Model file for the job. Use its own axes, mm. A direction names the side the tool comes from. Give positions to 0.01 mm unless a question says otherwise; leave off trailing zeros. Order: outer loops, then holes, each group sorted by start corner. A loop starts at its lowest first (then second) coordinate and runs counter-clockwise, first axis right, second up. Notation, with made-up numbers: M 82.5,-6.5 L 110.5,-6.5 A17 ccw 110.5,20.5 Z; hole C 72.5,85 d2. An arc over 180 degrees is marked long. Return JSON: item names as keys, results as strings. Group by question number.
1. Two-plate mould, pull along X, no slides. Class faces 4 (the face through (42.9, 3.4, 23.6)), 5 (the face through (1, 5, 0)), 6 (the face through (-44.45, 4.51, 22.3)): released by +X, released by -X, zero draft, split by the parting line, or undercut.
2. Slice it at C-C on z = 0. List the corners of the cut face in (x, y).
3. Wall check: probe 1 along X at (y, z) = (2.6, 25); probe 2 along Z at (x, y) = (-41.5, 3.65); probe 3 along X at (y, z) = (4.35, 25). Give the ranges that are in metal, low to high. Write a range as [from, to].
4. 3-axis set-ups, long thin cutter, end or side, ignore diameter. For faces 1 (the face through (40.979, 4.507, -28.966)), 2 (the face through (-38.327, 1.724, 25.705)), 3 (the face through (-29.084, 2.465, -2.703)): which of +Z, -Z, +X, -X, +Y, -Y reach the whole face in a straight line?
5. Slice it at A-A on z = 25. List the corners of the cut face in (x, y).
6. Slice it at D-D on y = 2.1. Give the number of separate pieces and of enclosed holes in the cut face, then the cut area to 3 significant figures.
7. Slice it at B-B on x = -20.5. List the corners of the cut face in (y, z).
8. Pin check, flat tips, straight feed: pin 1 (2 mm diameter, centred on x = -40.5, z = -24.5, fed in from -Y); pin 2 (7.5 mm diameter, centred on x = -41.5, z = 25, fed in from +Y). Stop position of each tip, or through.
Autodesk Inventor part; units mm, degrees
ref_plane "YZ Plane" through (0, 0, 0) normal (1, 0, 0) x (0, 1, 0)
ref_plane "XZ Plane" through (0, 0, 0) normal (0, 1, 0) x (-1, 0, 0)
ref_plane "XY Plane" through (0, 0, 0) normal (0, 0, 1) x (1, 0, 0)
sketch "Sketch1" plane through (0, 0, 0) normal (0, 1, 0) x (-1, 0, 0)
  line L0 (46.5, 30) -> (-46.5, 30)
  line L1 (-46.5, 30) -> (-46.5, -30)
  line L2 (-46.5, -30) -> (46.5, -30)
  line L3 (46.5, -30) -> (46.5, 30)
  line L4 (46.5, 30) -> (-46.5, -30) construction
  line L5 (-46.5, 30) -> (46.5, -30) construction
  circle A0 centre (20.5, 0) radius 9
  circle A1 centre (-19.5, 0) radius 12.5
  line L6 (152.1746, 0) -> (-152.1746, 0) construction
  line L7 (0, 58.0523) -> (0, -58.0523) construction
  point P0 (0, 0)
  dimension "d0" = 93
  dimension "d1" = 18
  dimension "d2" = 25
  dimension "d3" = 26
  dimension "d4" = 60
  dimension "d5" = 27
extrude "Extrusion1" add sketch "Sketch1" along normal blind 5
sketch "Sketch2" plane through (0, 0, 0) normal (0, -1, 0) x (1, 0, 0)
  line L0 (41.5, 25) -> (-41.5, 25) construction
  line L1 (-41.5, 25) -> (-41.5, -25) construction
  line L2 (-41.5, -25) -> (41.5, -25) construction
  line L3 (41.5, -25) -> (41.5, 25) construction
  line L4 (41.5, 25) -> (-41.5, -25) construction
  line L5 (-41.5, 25) -> (41.5, -25) construction
  line L6 (46.5, -30) -> (-46.5, -30) construction
  line L7 (-46.5, -30) -> (-46.5, 30) construction
  point P0 (0, 0)
  dimension "d11" = 5
  dimension "d12" = 5
hole "Hole1" at (41.5, 0, -25) at (-41.5, 0, -25) at (-41.5, 0, 25) at (41.5, 0, 25) direction (0, 1, 0) diameter 3.4 end through all counterbore diameter 6.5 counterbore depth 3.4
sketch "Sketch3" plane through (0, 5, 0) normal (0, 1, 0) x (1, 0, 0)
  circle A0 centre (-41.5, 25) radius 1.7
  circle A1 centre (-41.5, 25) radius 4
  circle A2 centre (41.5, -25) radius 1.7
  circle A3 centre (-41.5, -25) radius 1.7
  circle A4 centre (-41.5, 25) radius 1.7
  circle A5 centre (41.5, 25) radius 1.7
  line L0 (46.5, -30) -> (46.5, 30)
  line L1 (46.5, 30) -> (-46.5, 30)
  line L2 (-46.5, 30) -> (-46.5, -30)
  line L3 (-46.5, -30) -> (46.5, -30)
  circle A6 centre (41.5, 25) radius 4
  circle A7 centre (-41.5, -25) radius 4
  circle A8 centre (41.5, -25) radius 4
  point P0 (0, 0)
  dimension "d22" = 83
  dimension "d25" = 50
  dimension "d28" = 8
extrude "Extrusion2" cut sketch "Sketch3" against normal blind 1 contours A0 | A1 | A2 | A3 | A5 | A6 | A7 | A8
sketch "Sketch4" plane through (0, 5, 0) normal (0, 1, 0) x (1, 0, 0)
  circle A0 centre (41.5, -25) radius 4
  circle A1 centre (41.5, 25) radius 4
  circle A2 centre (-41.5, -25) radius 4
  circle A3 centre (-41.5, 25) radius 4
  line L0 (46.5, -30) -> (46.5, 30)
  line L1 (46.5, 30) -> (-46.5, 30)
  line L2 (-46.5, 30) -> (-46.5, -30)
  line L3 (-46.5, -30) -> (46.5, -30)
  circle A4 centre (-20.5, 0) radius 9
  circle A5 centre (19.5, 0) radius 12.5
  circle A6 centre (19.5, 0) radius 14
  point P0 (0, 0)
  dimension "d31" = 28
extrude "Extrusion3" cut sketch "Sketch4" against normal through all contours A6
sketch "Sketch6" plane through (0, 5, 0) normal (0, 1, 0) x (1, 0, 0)
  circle A0 centre (19.5, 0) radius 14
  circle A1 centre (19.5, 0) radius 21 construction
  line L0 (-65.1, 0) -> (65.1, 0)
  line L1 (19.5, 0) -> (9, -18.1865) construction
  point P0 (40.5, 0)
  point P1 (9, 18.1865)
  dimension "d40" = 42
  dimension "d43" = 360
  dimension "d66" = 60
hole "Hole2" at (40.5, 5, 0) at (9, 5, -18.1865) at (9, 5, 18.1865) direction (0, -1, 0) diameter 3.4 end through all
sketch "Sketch9" plane through (0, 0, 0) normal (0, -1, 0) x (1, 0, 0)
  circle A0 centre (19.5, 0) radius 12.5
  circle A1 centre (19.5, 0) radius 21 construction
  line L0 (-65.1, 0) -> (65.1, 0)
  line L1 (-1.5, 0) -> (19.5, 0) construction
  point P0 (0, 0)
  point P1 (30, 18.1865)
  point P2 (30, -18.1865)
  dimension "d53" = 42
  dimension "d63" = 360
hole "Hole3" at (30, 0, 18.1865) at (30, 0, -18.1865) direction (0, 1, 0) diameter 3 depth 4 tip angle 120
sketch "Sketch10" plane through (0, 5, 0) normal (0, 1, 0) x (1, 0, 0)
  circle A0 centre (19.5, 0) radius 14
  circle A1 centre (19.5, 0) radius 14.5
  point P0 (0, 0)
  dimension "d70" = 0.5
extrude "Extrusion5" cut sketch "Sketch10" against normal blind 0.25
properties part number "plate"
Result:
{
 "1": {"face 4": "undercut", "face 5": "zero draft", "face 6": "undercut"},
 "2": {"outline": "M -46.5,0 L -29.5,0 L -29.5,5 L -46.5,5 Z; M -11.5,0 L 5.5,0 L 5.5,4.75 L 5,4.75 L 5,5 L -11.5,5 Z; M 33.5,0 L 38.8,0 L 38.8,5 L 34,5 L 34,4.75 L 33.5,4.75 Z; M 42.2,0 L 46.5,0 L 46.5,5 L 42.2,5 Z"},
 "3": {"probe 1": "x = [-46.5, -44.75], [-38.25, 38.25], [44.75, 46.5]", "probe 2": "z = [-30, -26.7], [-23.3, 23.3], [26.7, 30]", "probe 3": "x = [-46.5, -45.5], [-37.5, 37.5], [45.5, 46.5]"},
 "4": {"face 1": "+Y", "face 2": "-Y", "face 3": "+Y, -Y"},
 "5": {"outline": "M -46.5,0 L -44.75,0 L -44.75,3.4 L -43.2,3.4 L -43.2,4 L -45.5,4 L -45.5,5 L -46.5,5 Z; M -39.8,3.4 L -38.25,3.4 L -38.25,0 L 38.25,0 L 38.25,3.4 L 39.8,3.4 L 39.8,4 L 37.5,4 L 37.5,5 L -37.5,5 L -37.5,4 L -39.8,4 Z; M 43.2,3.4 L 44.75,3.4 L 44.75,0 L 46.5,0 L 46.5,5 L 45.5,5 L 45.5,4 L 43.2,4 Z"},
 "6": {"separate pieces": "1", "enclosed holes": "11", "area": "4,540 mm2"},
 "7": {"outline": "M 0,-30 L 5,-30 L 5,-9 L 0,-9 Z; M 0,9 L 5,9 L 5,30 L 0,30 Z"},
 "8": {"pin 1": "stops at y = 3.4", "pin 2": "stops at y = 4"}
}
